The drawing under review shows one solid part. Ordinate dimensions are in mm from its lowest x, y, z. Round coordinates to 2 decimals unless told otherwise and drop trailing zeros. Write each loop counter-clockwise with the first axis right and the second up, starting at its lowest first coordinate (ties: lowest second). Pieces come first, ordered by that corner, then holes. Notation, with made-up numbers: M -37.5,68 L -4.5,68 A25 ccw -4.5,102 Z; hole C 39,-38 d9. An arc over 180 degrees is marked long. One line per item, written item: value. Start each with the question number.
1) Take a section at A-A, the plane x = 41. Write out the cut boundary in (y, z), and give its area (3 significant figures).
2) Mouldability with a two-part tool opening along Z and no side actions: class the marked faces 1, 2 and 3 as +Z half, -Z half, draft (parallel to the pull), parting line (faces both ways), or undercut.
3) Wall thickness on probe 1 along Z at (x, y) = (41, 10.75); probe 2 along Y at (x, z) = (24, 65); probe 3 along X at (y, z) = (6.25, 59): over which ranges is each line inside the solid? List them lowest first.
4) Take a section at B-B, the plane z = 51. Write out the cut boundary in (x, y).
5) For P1, Ø8, axis at y = 8, z = 65.5, coming from the +X side; P2, Ø3, axis at x = 81, y = 10.5, coming from the -Z side; P3, Ø6, axis at x = 39, y = 12, coming from the +Z side, all flat-tipped, find the tip position at first contact; note any pin that passes through.
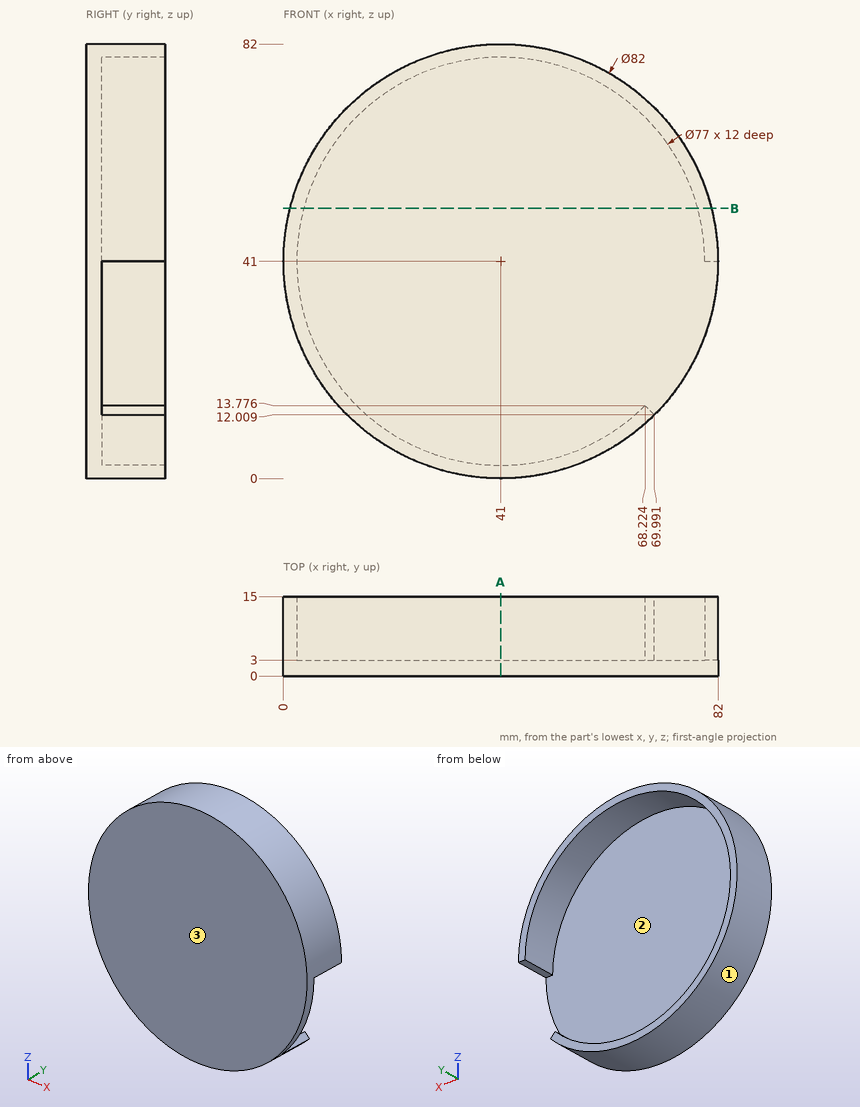
Checked values:
1. outline: M 0,0 L 15,0 L 15,2.5 L 3,2.5 L 3,79.5 L 15,79.5 L 15,82 L 0,82 Z
1. area: 306 mm2
2. face 1: parting line
2. face 2: undercut
2. face 3: draft
3. probe 1: z = 0 to 2.5, 79.5 to 82
3. probe 2: y = 0 to 3
3. probe 3: x = 4.16 to 6.97, 75.03 to 77.84
4. outline: M 1.24,0 L 80.76,0 L 80.76,15 L 78.18,15 L 78.18,3 L 3.82,3 L 3.82,15 L 1.24,15 Z
5. P1: stops at x = 76.51
5. P2: stops at z = 41
5. P3: stops at z = 82
